Geometry: final body of the model. Coordinates: model frame, mm. A direction names the side the tool comes from. Round coordinates to 2 decimals unless told otherwise and drop trailing zeros. Write each loop counter-clockwise with the first axis right and the second up, starting at its lowest first coordinate (ties: lowest second). Pieces come first, ordered by that corner, then holes. Notation, with made-up numbers: M 75.5,-15 L 108.5,-15 A21 cw 108.5,-7 Z; hole C -13.5,73.25 d3. An arc over 180 degrees is marked long. Put each result on its own line as item: value. Start each with the question number.
```python
from build123d import *

# Parameters (mm, degrees)
SKETCH2_W                  = 95
SKETCH2_H                  = 50
SKETCH2_W_2                = 80
SKETCH2_H_2                = 30
BOSS_EXTRUDE1_DEPTH        = 6
CUT_EXTRUDE1_DEPTH         = 55.011572834
CUT_EXTRUDE1_DEPTH_BACK    = 55.011572834
SKETCH4_R                  = 4
FILLET1_R                  = 10
M3X0_5_TAPPED_HOLE1_REACH  = 100.417
M3X0_5_TAPPED_HOLE1_BORE_R = 1.25
CHAMFER1_SIZE              = 10


with BuildPart() as part:
    # Sketch2 → Boss-Extrude1 (new, symmetric)
    with BuildSketch(Plane(origin=(0, 0, 0), x_dir=(1, 0, 0), z_dir=(0, 1, 0))):
        Rectangle(SKETCH2_W, SKETCH2_H)
        Rectangle(SKETCH2_W_2, SKETCH2_H_2, mode=Mode.SUBTRACT)
    extrude(amount=BOSS_EXTRUDE1_DEPTH, both=True)

    # Sketch4 → Cut-Extrude1 (cut, two sides: drawn at the far end of the back side and taken through both)
    with BuildSketch(Plane(origin=(0, 0, 0), x_dir=(0, 0, -1), z_dir=(1, 0, 0)).offset(-CUT_EXTRUDE1_DEPTH_BACK)):
        Circle(SKETCH4_R)
    extrude(amount=CUT_EXTRUDE1_DEPTH + CUT_EXTRUDE1_DEPTH_BACK, mode=Mode.SUBTRACT)

    # Fillet1
    fillet1_edges = [part.edges().sort_by_distance(p)[0] for p in [
        (40, 0, 15),
        (40, 0, -15),
        (-40, 0, -15),
        (-40, 0, 15),
    ]]
    fillet(fillet1_edges, radius=FILLET1_R)

    # M3x0.5 Tapped Hole1 bore → M3x0.5 Tapped Hole1 (cut, up to next)
    with BuildSketch(Plane.ZY.offset(47.5), mode=Mode.PRIVATE) as m3x0_5_tapped_hole1_sk1:
        with Locations((-9, 0)):
            Circle(M3X0_5_TAPPED_HOLE1_BORE_R)
    m3x0_5_tapped_hole1_tool1 = extrude(m3x0_5_tapped_hole1_sk1.sketch, amount=-M3X0_5_TAPPED_HOLE1_REACH, mode=Mode.PRIVATE) & part.part
    # M3x0.5 Tapped Hole1 bore → M3x0.5 Tapped Hole1 (cut, up to next)
    with BuildSketch(Plane.ZY.offset(47.5), mode=Mode.PRIVATE) as m3x0_5_tapped_hole1_sk2:
        with Locations((9, 0)):
            Circle(M3X0_5_TAPPED_HOLE1_BORE_R)
    m3x0_5_tapped_hole1_tool2 = extrude(m3x0_5_tapped_hole1_sk2.sketch, amount=-M3X0_5_TAPPED_HOLE1_REACH, mode=Mode.PRIVATE) & part.part
    m3x0_5_tapped_hole1_1 = m3x0_5_tapped_hole1_tool1.solids().sort_by_distance((-47.5, 0, -9))[0]
    add(m3x0_5_tapped_hole1_1, mode=Mode.SUBTRACT)
    m3x0_5_tapped_hole1_2 = m3x0_5_tapped_hole1_tool2.solids().sort_by_distance((-47.5, 0, 9))[0]
    add(m3x0_5_tapped_hole1_2, mode=Mode.SUBTRACT)
    m3x0_5_tapped_hole1 = m3x0_5_tapped_hole1_1 + m3x0_5_tapped_hole1_2  # M3x0.5 Tapped Hole1 as one shape, for the pattern or mirror that repeats it

    # Mirror1: M3x0.5 Tapped Hole1 across plane
    add(m3x0_5_tapped_hole1.mirror(Plane(origin=(0, 0, 0), x_dir=(0, 0, 1), z_dir=(1, 0, 0))), mode=Mode.SUBTRACT)

    # Hole Thread4: M3x0.5 Tapped Hole1 across Right Plane
    add(m3x0_5_tapped_hole1.mirror(Plane(origin=(0, 0, 0), x_dir=(0, 0, -1), z_dir=(1, 0, 0))), mode=Mode.SUBTRACT)

    # Chamfer1
    chamfer1_edges = [part.edges().sort_by_distance(p)[0] for p in [
        (47.5, 0, 25),
        (-47.5, 0, 25),
        (-47.5, 0, -25),
        (47.5, 0, -25),
    ]]
    chamfer(chamfer1_edges, length=CHAMFER1_SIZE)


solid = part.part
```
1) First-contact query: pin 1 (1 mm diameter, centred on x = -37.5, z = -6, fed in from +Y). Flat tip, straight axial feed; report the tip coordinate or a pass-through.
2) Section B-B, the plane z = -13. Output: boundary loops of the cut face in (x, y), and give its area (3 significant figures).
3) Draft query along Z for faces 1 (the face through (-36.99, 0.08, 12.15)), 2 (the face through (-47.5, 3, 4)), 3 (the face through (42.6, -0.1, 19.9)). Return one class per face: +Z half, -Z half, draft (parallel to the pull), parting line (faces both ways), or undercut.
4) Access query for faces 4 (the face through (-1, -6, -17)), 5 (the face through (-36.99, -0.08, -12.15)). Directions: +Z, -Z, +X, -X, +Y, -Y. A direction counts if a zero-diameter tool reaches every point of the face in a straight line with its end or side. Return the directions, or none.
5) Section A-A, the plane z = 0. Output: boundary loops of the cut face in (x, y).
6) Section C-C, the plane x = 6. Output: boundary loops of the cut face in (y, z).
7) Ray query, probe 1 along Z at (x, y) = (-7.5, -2.5); probe 2 along Z at (x, y) = (40.5, 0.25); probe 3 along Y at (x, z) = (-44.5, -9). Return the intervals inside material, ascending.
8) Section D-D, the plane y = 0. Give the number of separate pieces and of enclosed holes in the cut face, and give its area (3 significant figures).
Solved:
1. pin 1: passes through
2. outline: M -47.5,-6 L -36,-6 L -36,6 L -47.5,6 Z; M 36,-6 L 47.5,-6 L 47.5,6 L 36,6 Z
2. area: 276 mm2
3. face 1: undercut
3. face 2: draft
3. face 3: +Z half
4. face 4: +Z, -Z, +X, -X, -Y
4. face 5: +Y, -Y
5. outline: M -47.5,-6 L -40,-6 L -40,-4 L -47.5,-4 Z; M -47.5,4 L -40,4 L -40,6 L -47.5,6 Z; M 40,-6 L 47.5,-6 L 47.5,-4 L 40,-4 Z; M 40,4 L 47.5,4 L 47.5,6 L 40,6 Z
6. outline: M -6,-25 L 6,-25 L 6,-15 L -6,-15 Z; M -6,15 L 6,15 L 6,25 L -6,25 Z
7. probe 1: z = -25 to -15, 15 to 25
7. probe 2: z = -22 to -10.22, -7.78 to -3.99, 3.99 to 7.78, 10.22 to 22
7. probe 3: y = -6 to -1.25, 1.25 to 6
8. separate pieces: 6
8. enclosed holes: 0
8. area: 2,030 mm2
